Check sheet for the modelled part. Datum: model origin and axes. Units: mm. A direction names the side the tool comes from. Coordinates: 2 decimals unless noted, no trailing zeros. Write each loop counter-clockwise with the first axis right and the second up, starting at its lowest first coordinate (ties: lowest second). Pieces come first, ordered by that corner, then holes. Notation, with made-up numbers: (7, 37.25) -> (31, 37.25) arc R25 ccw to (31, 69.25) -> close; hole circle Ø2 at (29.25, 4.5). An arc over 180 degrees is marked (long way). Put each result on its own line as item: value.
```python
from build123d import *

# Parameters (mm, degrees)
SKETCH_1_W          = 28
SKETCH_1_H          = 35
SKETCH_1_R          = 2.1
SKETCH_1_R_2        = 6.505
EXTRUDE_1_DEPTH     = 6
CUT_EXTRUDE_1_DEPTH = 6
FILLET_1_R          = 1
CUT_EXTRUDE_2_DEPTH = 10
FILLET_2_R          = 3


with BuildPart() as part:
    # 草图1 → 凸台-拉伸1 (new body)
    with BuildSketch(Plane(origin=(0, 0, 0), x_dir=(1, 0, 0), z_dir=(0, 1, 0))):
        Rectangle(SKETCH_1_W, SKETCH_1_H)
        with Locations(Location((9.5, 11.5, 0), (0, 0, 270))):
            Circle(SKETCH_1_R, mode=Mode.SUBTRACT)
        with Locations(Location((9.5, -11.5, 0), (0, 0, 270))):
            Circle(SKETCH_1_R, mode=Mode.SUBTRACT)
        with Locations(Location((-2.5, 0, 0), (0, 0, 270))):
            Circle(SKETCH_1_R_2, mode=Mode.SUBTRACT)
    extrude(amount=EXTRUDE_1_DEPTH)

    # 草图2 → 切除-拉伸1 (cut)
    with BuildSketch(Plane(origin=(0, 6, 0), x_dir=(1, 0, 0), z_dir=(0, 1, 0))):
        Polygon((14, 12.5), (13, 11.5), (13, -11.5), (14, -12.5), align=None)
    extrude(amount=-CUT_EXTRUDE_1_DEPTH, mode=Mode.SUBTRACT)

    # 圆角1
    fillet_1_edges = [part.edges().sort_by_distance(p)[0] for p in [
        (13, 3, 11.5),
        (13, 3, -11.5),
        (14, 3, -12.5),
        (14, 3, 12.5),
    ]]
    fillet(fillet_1_edges, radius=FILLET_1_R)

    # 草图3 → 切除-拉伸2 (cut)
    with BuildSketch(Plane(origin=(0, 6, 0), x_dir=(1, 0, 0), z_dir=(0, 1, 0))):
        with BuildLine():
            Line((-14, -17.5), (-6, -17.5))
            Line((-6, -17.5), (-12.576618502, -5.541819157))
            ThreePointArc((-12.576618502, -5.541819157), (-13.638471902, -2.860846674), (-14, -2.8e-08))
            Line((-14, -2.8e-08), (-14, -17.5))
        make_face()
        with BuildLine():
            Line((-14, 17.5), (-14, -2.8e-08))
            ThreePointArc((-14, -2.8e-08), (-13.638471909, 2.860846647), (-12.576618502, 5.541819157))
            Line((-12.576618502, 5.541819157), (-6, 17.5))
            Line((-6, 17.5), (-14, 17.5))
        make_face()
    extrude(amount=-CUT_EXTRUDE_2_DEPTH, mode=Mode.SUBTRACT)

    # 圆角2
    fillet_2_edges = [part.edges().sort_by_distance(p)[0] for p in [
        (-6, 3, 17.5),
        (14, 3, 17.5),
        (14, 3, -17.5),
        (-6, 3, -17.5),
    ]]
    fillet(fillet_2_edges, radius=FILLET_2_R)


solid = part.part
```
Q1. Cross-section at A-A (x = 9.5). Record the cut outline in (y, z).
Recorded:
outline: (0, -17.5) -> (6, -17.5) -> (6, -13.6) -> (0, -13.6) -> close; (0, -9.4) -> (6, -9.4) -> (6, 9.4) -> (0, 9.4) -> close; (0, 13.6) -> (6, 13.6) -> (6, 17.5) -> (0, 17.5) -> close
Q2. Material ranges on line 1 along Z through (x, y) = (7.75, 3.4); line 2 along X through (y, z) = (4.6, 5.5); line 3 along X through (y, z) = (2.3, -11), recorded low to high.
Recorded:
line 1: z = -17.5 to -12.66, -10.34 to 10.34, 12.66 to 17.5
line 2: x = -12.6 to -5.97, 0.97 to 13
line 3: x = -9.57 to 7.46, 11.54 to 13
Q3. Cross-section at B-B (y = 0.5). Record the cut outline in (x, z) (3 decimals), plus the area to 3 significant figures.
Recorded:
outline: (-12.577, -5.542) -> (-6.855, -15.946) arc R3 ccw to (-4.226, -17.5) -> (11, -17.5) arc R3 ccw to (14, -14.5) -> (14, -12.914) arc R1 ccw to (13.707, -12.207) -> (13.293, -11.793) arc R1 cw to (13, -11.086) -> (13, 11.086) arc R1 cw to (13.293, 11.793) -> (13.707, 12.207) arc R1 ccw to (14, 12.914) -> (14, 14.5) arc R3 ccw to (11, 17.5) -> (-4.226, 17.5) arc R3 ccw to (-6.855, 15.946) -> (-12.577, 5.542) arc R11.5 ccw to start; hole circle Ø13.01 at (-2.5, 0); hole circle Ø4.2 at (9.5, -11.5); hole circle Ø4.2 at (9.5, 11.5)
area: 673 mm2
Q4. Depth check by flat-ended pin: P1, Ø1.5, axis at x = -6.5, y = 4, coming from the +Z side. Enter the tip coordinate at first touch or a pass-through.
Recorded:
P1: stops at z = 17.08
Q5. Cross-section at D-D (z = 1). Record the cut outline in (x, y), plus the area to 3 significant figures.
Recorded:
outline: (-13.96, 0) -> (-8.93, 0) -> (-8.93, 6) -> (-13.96, 6) -> close; (3.93, 0) -> (13, 0) -> (13, 6) -> (3.93, 6) -> close
area: 84.6 mm2
Q6. Tool access check on faces 1 (the flat face through (13, 3, 0)), 2 (the flat face through (14, 3, 14)). Record the directions out of +Z, -Z, +X, -X, +Y, -Y that give a thin tool (end or side, any length) a straight path to the whole face; none if there is none.
Recorded:
face 1: +X, +Y, -Y
face 2: +Z, -Z, +X, +Y, -Y
Q7. Cross-section at C-C (x = -2.5). Record the cut outline in (y, z) (3 decimals), plus the area to 3 significant figures.
Recorded:
outline: (0, -17.5) -> (6, -17.5) -> (6, -6.505) -> (0, -6.505) -> close; (0, 6.505) -> (6, 6.505) -> (6, 17.5) -> (0, 17.5) -> close
area: 132 mm2
Q8. Mould release check, pull along Z, two halves, no side actions. Record for faces 3 (the cylindrical face through (10.919, 2.958, -13.048)), 4 (the cylindrical face through (-5.77, 2.96, -17.07)), 5 (the cylindrical face through (1.9, 2.96, -4.79)), 6 (the flat face through (3, 3, 17.5)): released by +Z, released by -Z, zero draft, split by the parting line, or undercut.
Recorded:
face 3: undercut
face 4: released by -Z
face 5: undercut
face 6: released by +Z
